CAD build for the part. Positions are in the model's coordinates, mm. A direction names the side the tool comes from. Give positions to 0.01 mm unless a question says otherwise; leave off trailing zeros. Write each loop counter-clockwise with the first axis right and the second up, starting at its lowest first coordinate (ties: lowest second). Pieces come first, ordered by that corner, then holes. Notation, with made-up numbers: (31, 77.5) - (79, 77.5) arc R22 ccw to (79, 98.5) - close; hole circle Ø10 at (60, 81). An arc over 180 degrees is marked (long way). Answer as a JSON object with one key per item and string values.
from build123d import *

# Parameters (mm, degrees)
ESQUISSE1_W             = 35
ESQUISSE1_H             = 31
ESQUISSE1_R             = 1.6
ESQUISSE1_R_2           = 5
BOSS_EXTRU_1_DEPTH      = 1.5
ESQUISSE2_W             = 35
ESQUISSE2_H             = 1.5
BOSS_EXTRU_2_DEPTH      = 40
ENL_V_MAT_EXTRU_1_DEPTH = 32.5
ESQUISSE4_R             = 9
ESQUISSE4_R_2           = 1.15
ENL_V_MAT_EXTRU_2_DEPTH = 32.5


with BuildPart() as part:
    # Esquisse1 → Boss.-Extru.1 (new body)
    with BuildSketch(Plane(origin=(0, 0, 0), x_dir=(1, 0, 0), z_dir=(0, 1, 0))):
        Rectangle(ESQUISSE1_W, ESQUISSE1_H)
        with Locations(Location((-10.480234522, 9.282493434, 0), (0, 0, 270))):
            Circle(ESQUISSE1_R, mode=Mode.SUBTRACT)
        with Locations(Location((0, 0, 0), (0, 0, 270))):
            Circle(ESQUISSE1_R_2, mode=Mode.SUBTRACT)
        with Locations(Location((10.480234522, 9.282493434, 0), (0, 0, 90))):
            Circle(ESQUISSE1_R, mode=Mode.SUBTRACT)
        with Locations(Location((10.480234522, -9.282493434, 0), (0, 0, 270))):
            Circle(ESQUISSE1_R, mode=Mode.SUBTRACT)
        with Locations(Location((-10.480234522, -9.282493434, 0), (0, 0, 90))):
            Circle(ESQUISSE1_R, mode=Mode.SUBTRACT)
    extrude(amount=BOSS_EXTRU_1_DEPTH)

    # Esquisse2 → Boss.-Extru.2 (add)
    with BuildSketch(Plane(origin=(0, 1.5, 0), x_dir=(1, 0, 0), z_dir=(0, 1, 0))):
        with Locations((0, -14.75)):
            Rectangle(ESQUISSE2_W, ESQUISSE2_H)
    extrude(amount=BOSS_EXTRU_2_DEPTH)

    # Esquisse3 → Enlèv. mat.-Extru.1 (cut)
    with BuildSketch(Plane.XY.offset(15.5)):
        with BuildLine():
            Line((-17.5, 41.5), (-17.5, 28))
            ThreePointArc((-17.5, 28), (-15.829114832, 35.462514566), (-11.135528726, 41.5))
            Line((-11.135528726, 41.5), (-17.5, 41.5))
        make_face()
        with BuildLine():
            Line((17.5, 41.5), (11.135528726, 41.5))
            ThreePointArc((11.135528726, 41.5), (15.829114832, 35.462514566), (17.5, 28))
            Line((17.5, 28), (17.5, 41.5))
        make_face()
    extrude(amount=-ENL_V_MAT_EXTRU_1_DEPTH, mode=Mode.SUBTRACT)

    # Esquisse4 → Enlèv. mat.-Extru.2 (cut)
    with BuildSketch(Plane.XY.offset(15.5)):
        with Locations((0, 28)):
            Circle(ESQUISSE4_R)
        with Locations((-15, 28)):
            Circle(ESQUISSE4_R_2)
        with Locations((15, 28)):
            Circle(ESQUISSE4_R_2)
    extrude(amount=-ENL_V_MAT_EXTRU_2_DEPTH, mode=Mode.SUBTRACT)


solid = part.part
(1) Flat gauge pins, fed straight in: P1, Ø20.5, axis at x = 0, y = 28, coming from the -Z side; P2, Ø1.9, axis at x = 10.48, z = -9.28, coming from the -Y side; P3, Ø5, axis at x = -10.48, z = -9.28, coming from the -Y side; P4, Ø5, axis at x = -10.48, z = 9.28, coming from the +Y side. Where does each tip first touch, or does it go through?
Answer key:
{"P1": "stops at z = 14", "P2": "passes through", "P3": "stops at y = 0", "P4": "stops at y = 1.5"}
(2) 3-axis set-ups, long thin cutter, end or side, ignore diameter. For faces 4 (the face through (17.5, 1, 5)), 5 (the face through (0, 17, 14)): which of +Z, -Z, +X, -X, +Y, -Y reach the whole face in a straight line?
Answer key:
{"face 4": "+Z, -Z, +X, +Y, -Y", "face 5": "-Z, +X, -X, +Y"}
(3) Saw through at B-B, the plane z = 0. Give the cut face in (x, y), and give its area (3 significant figures).
Answer key:
{"outline": "(-17.5, 0) - (-5, 0) - (-5, 1.5) - (-17.5, 1.5) - close; (5, 0) - (17.5, 0) - (17.5, 1.5) - (5, 1.5) - close", "area": "37.5 mm²"}
(4) Saw through at A-A, the plane x = 0. Give the cut face in (y, z).
Answer key:
{"outline": "(0, -15.5) - (1.5, -15.5) - (1.5, -5) - (0, -5) - close; (0, 5) - (1.5, 5) - (1.5, 14) - (19, 14) - (19, 15.5) - (0, 15.5) - close; (37, 14) - (41.5, 14) - (41.5, 15.5) - (37, 15.5) - close"}
(5) Saw through at C-C, the plane y = 36. Give the cut face in (x, z).
Answer key:
{"outline": "(-15.56, 14) - (-4.12, 14) - (-4.12, 15.5) - (-15.56, 15.5) - close; (4.12, 14) - (15.56, 14) - (15.56, 15.5) - (4.12, 15.5) - close"}
(6) Saw through at D-D, the plane x = 8. Give the cut face in (y, z).
Answer key:
{"outline": "(0, -15.5) - (1.5, -15.5) - (1.5, 14) - (23.88, 14) - (23.88, 15.5) - (0, 15.5) - close; (32.12, 14) - (41.5, 14) - (41.5, 15.5) - (32.12, 15.5) - close"}
(7) Probe L1, parallel to Y at x = 0, z = 15.1; L2, parallel to X at y = 1.15, z = 0; L3, parallel to Y at x = -12, z = 13. List the from-to ranges inside material, lowest first. Write a range as [from, to].
Answer key:
{"L1": "y = [0, 19], [37, 41.5]", "L2": "x = [-17.5, -5], [5, 17.5]", "L3": "y = [0, 1.5]"}
(8) Pull direction Y, two halves, no side cores. Call faces 1 (the face through (-15.249, 26.877, 14.76)), 2 (the face through (0, 1, -15.5)), 3 (the face through (4, 1.5, -4)): pulls with the +Y half, pulls with the -Y half, needs draft (parallel to the pull), parting line crosses it, or undercut.
Answer key:
{"face 1": "undercut", "face 2": "needs draft", "face 3": "pulls with the +Y half"}
